Input: part model. Units: mm. Frame: model coordinates. Round coordinates to 2 decimals unless told otherwise and drop trailing zeros. Order: outer loops, then holes, each group sorted by start corner. A loop starts at its lowest first (then second) coordinate and runs counter-clockwise, first axis right, second up. Notation, with made-up numbers: (-22, 21) -> (-15, 21) arc R18 cw to (-15, 49) -> close; hole circle Ø6 at (64.25, 21.5). An arc over 180 degrees is marked (long way). Answer as CSV lines item,"result". Start each with the question number.
1) Line query: L1, parallel to X at y = 16.5, z = 0.4 (3 decimals); L2, parallel to X at y = 13.5, z = 0.55; L3, parallel to X at y = 5.5, z = 0.45. Output: solid intervals per line, ascending.
2) Section query B-B, the plane y = 24. Output: boundary loops of the cut face in (x, z).
3) Section query C-C, the plane z = 0.8. Output: boundary loops of the cut face in (x, y), and give its area (3 significant figures).
4) Section query A-A, the plane x = -12. Output: boundary loops of the cut face in (y, z), and give its area (3 significant figures).
5) Section query D-D, the plane y = -11. Output: boundary loops of the cut face in (x, z), and give its area (3 significant figures).
```python
from build123d import *

# Parameters (mm, degrees)
SKETCH1_R           = 25
SKETCH1_R_2         = 2.2
SKETCH1_R_3         = 3.15
BOSS_EXTRUDE1_DEPTH = 1.5


with BuildPart() as part:
    # Sketch1 → Boss-Extrude1 (new body)
    with BuildSketch(Plane.XY):
        with Locations((-2.056478496, 7.394811009)):
            Circle(SKETCH1_R)
        with Locations((-2.056478496, -12.605188991)):
            Circle(SKETCH1_R_2, mode=Mode.SUBTRACT)
        with Locations((-2.056478496, 7.394811009)):
            Circle(SKETCH1_R_3, mode=Mode.SUBTRACT)
        with BuildLine():
            ThreePointArc((19.743521504, 7.394811009), (-2.256478496, 29.594811009), (-24.256478496, 7.394811009))
            ThreePointArc((-24.256478496, 7.394811009), (-22.056478496, 5.194811009), (-19.856478496, 7.394811009))
            ThreePointArc((-19.856478496, 7.394811009), (-2.256478496, 25.194811009), (15.343521504, 7.394811009))
            ThreePointArc((15.343521504, 7.394811009), (17.543521504, 5.194811009), (19.743521504, 7.394811009))
        make_face(mode=Mode.SUBTRACT)
    extrude(amount=BOSS_EXTRUDE1_DEPTH)


solid = part.part
```
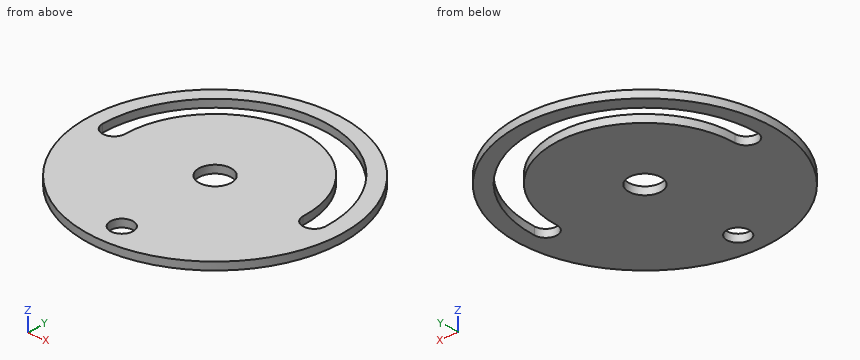
Findings:
1,L1,"x = -25.339 to -22.374, -17.438 to 12.925, 17.861 to 21.226"
1,L2,"x = -26.3 to -23.45, -18.84 to 14.32, 18.94 to 22.19"
1,L3,"x = -26.98 to -23.17, -20.94 to -4.57, 0.46 to 16.43, 18.66 to 22.87"
2,outline,"(-20.75, 0) -> (-16.92, 0) -> (-16.92, 1.5) -> (-20.75, 1.5) -> close; (-8.63, 0) -> (4.12, 0) -> (4.12, 1.5) -> (-8.63, 1.5) -> close; (12.4, 0) -> (16.63, 0) -> (16.63, 1.5) -> (12.4, 1.5) -> close"
3,outline,"circle Ø50 at (-2.06, 7.39); hole (-24.26, 7.39) arc R2.2 ccw to (-19.86, 7.39) arc R17.6 cw (long way) to (15.34, 7.39) arc R2.2 ccw to (19.74, 7.39) arc R22 ccw (long way) to start; hole circle Ø6.3 at (-2.06, 7.39); hole circle Ø4.4 at (-2.06, -12.61)"
3,area,"1,630 mm^2"
4,outline,"(-15.54, 0) -> (22.25, 0) -> (22.25, 1.5) -> (-15.54, 1.5) -> close; (27.32, 0) -> (30.33, 0) -> (30.33, 1.5) -> (27.32, 1.5) -> close"
4,area,"61.2 mm^2"
5,outline,"(-18.99, 0) -> (-3.56, 0) -> (-3.56, 1.5) -> (-18.99, 1.5) -> close; (-0.55, 0) -> (14.87, 0) -> (14.87, 1.5) -> (-0.55, 1.5) -> close"
5,area,"46.3 mm^2"
